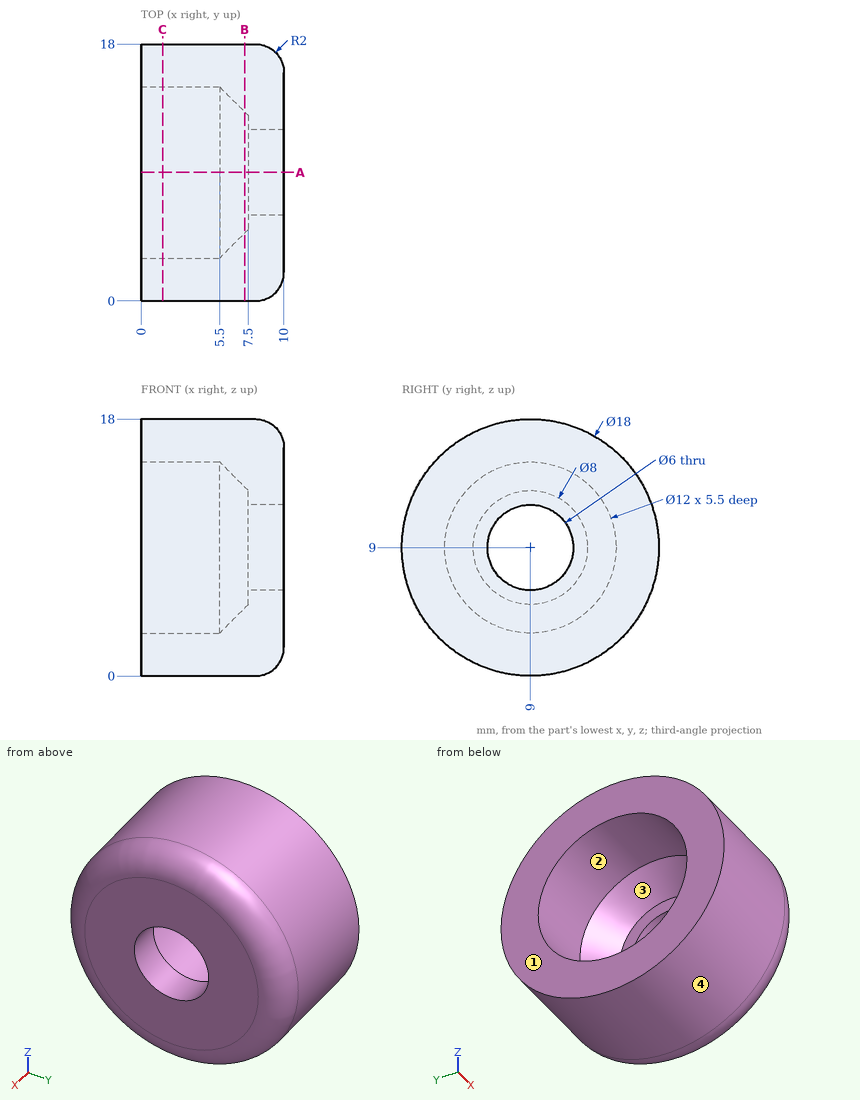
Answer from the drawing. Dimensions are ordinates in mm from the lowest x, y and z of the part. Round coordinates to 2 decimals unless told otherwise and drop trailing zeros. Write each loop counter-clockwise with the first axis right and the second up, starting at its lowest first coordinate (ties: lowest second). Pieces come first, ordered by that corner, then holes. Notation, with made-up numbers: (-12, -4.5) - (46, -4.5) arc R28 ccw to (46, 21.5) - close; hole circle Ø4 at (-5, 27). An arc over 180 degrees is marked (long way). Use a Markdown table: item, result.
(1) The mould has two halves that part along Y. Classify the marked faces 1, 2, 3 and 4: released by +Y, released by -Y, zero draft, split by the parting line, or undercut.
Reported:
| item | result |
|---|---|
| face 1 | zero draft |
| face 2 | undercut |
| face 3 | undercut |
| face 4 | split by the parting line |
(2) Each of these flat-tipped pins is pushed along its axis until it touches: pin 1 Ø4 at (x, y) = (9, 5.5) entering from -Z; pin 2 Ø6.5 at (y, z) = (8, 8.5) entering from -X; pin 3 Ø5 at (x, z) = (4.5, 2) entering from -Y. Where does it stop, or does it pass through?
Reported:
| item | result |
|---|---|
| pin 1 | z = 0.17 |
| pin 2 | x = 7.13 |
| pin 3 | y = 1.21 |
(3) The part is cut by section A-A (y = 9). Write down the section's boundary in (x, z).
Reported:
| item | result |
|---|---|
| outline | (0, 0) - (8, 0) arc R2 ccw to (10, 2) - (10, 6) - (7.5, 6) - (7.5, 5) - (5.5, 3) - (0, 3) - close; (0, 15) - (5.5, 15) - (7.5, 13) - (7.5, 12) - (10, 12) - (10, 16) arc R2 ccw to (8, 18) - (0, 18) - close |
(4) Straight lines are drawn through the part: line 1 along Z through (x, y) = (4, 4.5); line 2 along Z through (x, y) = (1.3, 9); line 3 along X through (y, z) = (6.5, 11.25). For each, find the intervals that lie inside material, in ascending order. Write a range as [from, to].
Reported:
| item | result |
|---|---|
| line 1 | [1.21, 5.03], [12.97, 16.79] |
| line 2 | [0, 3], [15, 18] |
| line 3 | [7.5, 10] |
(5) The part is cut by section C-C (x = 1.5). Write down the section's boundary in (y, z), then the cut area to 3 significant figures.
Reported:
| item | result |
|---|---|
| outline | circle Ø18 at (9, 9); hole circle Ø12 at (9, 9) |
| area | 141 mm2 |
(6) The part is cut by section B-B (x = 7.25). Write down the section's boundary in (y, z).
Reported:
| item | result |
|---|---|
| outline | circle Ø18 at (9, 9); hole circle Ø8.5 at (9, 9) |
